```python
from build123d import *

# Parameters (mm, degrees)
SKETCH1_W                                            = 76.2
SKETCH1_H                                            = 88.9
BOSS_EXTRUDE1_DEPTH                                  = 6.35
CSK_FOR_2_FLAT_HEAD_SOCKET_CAP_SCREW1_D              = 2.4384
CSK_FOR_2_FLAT_HEAD_SOCKET_CAP_SCREW1_DEPTH          = 6.4
CSK_FOR_2_FLAT_HEAD_SOCKET_CAP_SCREW1_CSINK_D        = 5.0038
CSK_FOR_2_FLAT_HEAD_SOCKET_CAP_SCREW1_CSINK_ANGLE    = 82
CSK_FOR_2_FLAT_HEAD_SOCKET_CAP_SCREW1_TIP            = 0.732569267
CBORE_FOR_1_4_BINDING_HEAD_MACHINE_SCREW_D           = 6.7564
CBORE_FOR_1_4_BINDING_HEAD_MACHINE_SCREW_DEPTH       = 6.4
CBORE_FOR_1_4_BINDING_HEAD_MACHINE_SCREW_CBORE_D     = 14.2875
CBORE_FOR_1_4_BINDING_HEAD_MACHINE_SCREW_CBORE_DEPTH = 4.191
CBORE_FOR_1_4_BINDING_HEAD_MACHINE_SCREW_TIP         = 2.029827343


with BuildPart() as part:
    # Sketch1 → Boss-Extrude1 (new body)
    with BuildSketch(Plane(origin=(0, 0, 0), x_dir=(1, 0, 0), z_dir=(0, 1, 0))):
        with Locations((38.1, 44.45)):
            Rectangle(SKETCH1_W, SKETCH1_H)
    extrude(amount=BOSS_EXTRUDE1_DEPTH)

    # CSK for #2 Flat Head Socket Cap Screw1
    with Locations(Plane(origin=(0, 6.35, 0), x_dir=(1, 0, 0), z_dir=(0, 1, 0))):
        with Locations((33.6, 20.9), (30.1, 53.9)):
            CounterSinkHole(CSK_FOR_2_FLAT_HEAD_SOCKET_CAP_SCREW1_D / 2, CSK_FOR_2_FLAT_HEAD_SOCKET_CAP_SCREW1_CSINK_D / 2, depth=CSK_FOR_2_FLAT_HEAD_SOCKET_CAP_SCREW1_DEPTH, counter_sink_angle=CSK_FOR_2_FLAT_HEAD_SOCKET_CAP_SCREW1_CSINK_ANGLE)
            with Locations((0, 0, -(CSK_FOR_2_FLAT_HEAD_SOCKET_CAP_SCREW1_DEPTH + CSK_FOR_2_FLAT_HEAD_SOCKET_CAP_SCREW1_TIP / 2))):  # 118° drill point
                Cone(0, CSK_FOR_2_FLAT_HEAD_SOCKET_CAP_SCREW1_D / 2, CSK_FOR_2_FLAT_HEAD_SOCKET_CAP_SCREW1_TIP, mode=Mode.SUBTRACT)

    # CBORE for 1/4 Binding Head Machine Screw1
    with Locations(Plane(origin=(0, 0, 0), x_dir=(-1, 0, 0), z_dir=(0, -1, 0))):
        with Locations((-63.0936, 44.45), (-13.1064, 31.9532), (-13.1064, 56.9468)):
            CounterBoreHole(CBORE_FOR_1_4_BINDING_HEAD_MACHINE_SCREW_D / 2, CBORE_FOR_1_4_BINDING_HEAD_MACHINE_SCREW_CBORE_D / 2, CBORE_FOR_1_4_BINDING_HEAD_MACHINE_SCREW_CBORE_DEPTH, depth=CBORE_FOR_1_4_BINDING_HEAD_MACHINE_SCREW_DEPTH)
            with Locations((0, 0, -(CBORE_FOR_1_4_BINDING_HEAD_MACHINE_SCREW_DEPTH + CBORE_FOR_1_4_BINDING_HEAD_MACHINE_SCREW_TIP / 2))):  # 118° drill point
                Cone(0, CBORE_FOR_1_4_BINDING_HEAD_MACHINE_SCREW_D / 2, CBORE_FOR_1_4_BINDING_HEAD_MACHINE_SCREW_TIP, mode=Mode.SUBTRACT)


solid = part.part
```
Work out the finished part from the listing and answer in its coordinate system (mm). A direction names the side the tool comes from. Give positions to 0.01 mm unless a question says otherwise; leave off trailing zeros. Order: outer loops, then holes, each group sorted by start corner. A loop starts at its lowest first (then second) coordinate and runs counter-clockwise, first axis right, second up.
1. The mould has two halves that part along X. Classify faces 3 (the flat face through (76.2, 3, -44)), 4 (the flat face through (62, 4.191, -41)), 5 (the flat face through (38, 3, -88.9)): released by +X, released by -X, zero draft, split by the parting line, or undercut.
Result sheet:
face 3: released by +X
face 4: undercut
face 5: zero draft
2. Straight lines are drawn through the part: L1, parallel to Z at x = 30.1, y = 3.7; L2, parallel to Z at x = 7.5, y = 1.5; L3, parallel to Z at x = 15, y = 3.5. For each, find the intervals that lie inside material, in ascending order.
Result sheet:
L1: z = -88.9 to -55.12, -52.68 to 0
L2: z = -88.9 to -61.37, -52.52 to -36.38, -27.53 to 0
L3: z = -88.9 to -63.84, -50.06 to -38.84, -25.06 to 0
3. Section B-B, the plane z = -33.5 is taken. Determine the outline of the cut face in (x, y), and give its area (3 significant figures).
Result sheet:
outline: (0, 0) - (6.13, 0) - (6.13, 4.19) - (10.1, 4.19) - (10.1, 6.35) - (0, 6.35) - close; (16.11, 4.19) - (20.08, 4.19) - (20.08, 0) - (76.2, 0) - (76.2, 6.35) - (16.11, 6.35) - close
area: 412 mm2
4. Each of these flat-tipped pins is pushed along its axis until it touches: P1, Ø5.5, axis at x = 63.09, z = -44.45, coming from the +Y side; P2, Ø4.5, axis at x = 61.5, z = -41, coming from the -Y side; P3, Ø3, axis at x = 33.6, z = -20.9, coming from the +Y side. Where does it stop, or does it pass through?
Result sheet:
P1: passes through
P2: stops at y = 4.19
P3: stops at y = 5.2
5. For faces 1 (the cylindrical face through (14.036, 2.066, -39.036)), 2 (the cylindrical face through (34.82, 2.4, -20.95)), determine the directions among +Z, -Z, +X, -X, +Y, -Y from which every point of the face is accessible in a straight line to the end or side of a thin tool.
Result sheet:
face 1: -Y
face 2: +Y, -Y
6. Section D-D, the plane x = 68.5 is taken. Determine the outline of the cut face in (y, z), and give its area (3 significant figures).
Result sheet:
outline: (0, -88.9) - (6.35, -88.9) - (6.35, 0) - (0, 0) - (0, -39.78) - (4.19, -39.78) - (4.19, -49.12) - (0, -49.12) - close
area: 525 mm2
7. Section C-C, the plane y = 1 is taken. Determine the outline of the cut face in (x, z), and give its area (3 significant figures).
Result sheet:
outline: (0, -88.9) - (76.2, -88.9) - (76.2, 0) - (0, 0) - close; hole circle Ø14.29 at (13.11, -56.95); hole circle Ø14.29 at (13.11, -31.95); hole circle Ø2.44 at (30.1, -53.9); hole circle Ø2.44 at (33.6, -20.9); hole circle Ø14.29 at (63.09, -44.45)
area: 6,280 mm2
8. Section A-A, the plane x = 33.6 is taken. Determine the outline of the cut face in (y, z).
Result sheet:
outline: (0, -88.9) - (6.35, -88.9) - (6.35, -23.4) - (4.87, -22.12) - (0, -22.12) - close; (0, -19.68) - (4.87, -19.68) - (6.35, -18.4) - (6.35, 0) - (0, 0) - close
